```python
from build123d import *

# Parameters (mm, degrees)
F2_DEPTH = 100
F3_W     = 86
F3_H     = 92
F4_DEPTH = 3


# Not quite as in the source:
# - the program builds the solid bodies; features that only make, move or delete a surface that nothing else refers to are left out


with BuildPart() as f2:
    # F0 (on Top) → F2 (new body)
    with BuildSketch(Plane.XY):
        Polygon((-2.3052925244, 0), (87.6947074756, 0), (87.6947074756, 8), (85.6947074756, 8), (85.6947074756, 3), (-0.3052925244, 3), (-0.3052925244, 11), (-59.3052925244, 11), (-59.3052925244, 8), (-2.3052925244, 8), (-2.3052925244, 3), align=None)
    extrude(amount=-F2_DEPTH)

    # F3 (on Front) → F4 (cut)
    with BuildSketch(Plane.XZ):
        with Locations((42.6947074756, -50)):
            Rectangle(F3_W, F3_H)
    extrude(amount=-F4_DEPTH, mode=Mode.SUBTRACT)


solid = f2.part
```
Source: CAD feature listing. Evaluate the final solid. Frame: model axes, mm. A direction names the side the tool comes from. Round coordinates to 2 decimals unless told otherwise and drop trailing zeros. Write each loop counter-clockwise with the first axis right and the second up, starting at its lowest first coordinate (ties: lowest second). Pieces come first, ordered by that corner, then holes. Notation, with made-up numbers: M -25.75,-24 L -2.75,-24 A15 ccw -2.75,-17 Z; hole C 44,8 d6. An arc over 180 degrees is marked long. Answer as a JSON object with one key per item and string values. Group by question number.
(1) Ray query, line 1 (X direction, y = 1.5, z = -17); line 2 (X direction, y = 10.5, z = -64); line 3 (Y direction, x = -12.5, z = -81). Return the intervals inside material, ascending. Write a range as [from, to].
(2) Section query C-C on x = 40. Output: boundary loops of the cut face in (y, z).
(3) Mould query, pull axis Z, two halves, no side actions, for faces 1 (the flat face through (42, 1, -96)), 2 (the flat face through (13.9, 2.7, 0)), 3 (the flat face through (-31, 8, -49)). Classes: +Z half, -Z half, draft (parallel to the pull), parting line (faces both ways), or undercut.
(4) Section query A-A on z = -15.5. Output: boundary loops of the cut face in (x, y).
(5) First-contact query: pin 1 (5 mm diameter, centred on x = -35.5, y = 3.5, fed in from -Z); pin 2 (1.2 mm diameter, centred on x = 45, z = -3, fed in from +Y); pin 3 (1.6 mm diameter, centred on x = 87, z = -26, fed in from +Y); pin 4 (6.5 mm diameter, centred on y = 3, z = -52, fed in from -X). Flat tips, straight axial feed; report the tip coordinate or a pass-through.
(6) Section query D-D on x = -7. Output: boundary loops of the cut face in (y, z), then the cut area to 3 significant figures.
(7) Reachability of faces 4 (the flat face through (-29, 11, -49)), 5 (the flat face through (-2.305, 4, -49)), 6 (the flat face through (43, 3, -98)), 7 (the flat face through (87.695, 4, -49)), 8 (the flat face through (42, 1, -4)) from +Z, -Z, +X, -X, +Y, -Y: full face, straight path, thin tool, end or side. Return the list, or none.
(8) Section query B-B on y = 6.25. Output: boundary loops of the cut face in (x, z), then the cut area to 3 significant figures.
Computed values:
{
 "1": {"line 1": "[-2.31, -0.31], [85.69, 87.69]", "line 2": "[-59.31, -0.31]", "line 3": "[8, 11]"},
 "2": {"outline": "M 0,-100 L 3,-100 L 3,-96 L 0,-96 Z; M 0,-4 L 3,-4 L 3,0 L 0,0 Z"},
 "3": {"face 1": "undercut", "face 2": "+Z half", "face 3": "draft"},
 "4": {"outline": "M -59.31,8 L -2.31,8 L -2.31,0 L -0.31,0 L -0.31,11 L -59.31,11 Z; M 85.69,0 L 87.69,0 L 87.69,8 L 85.69,8 Z"},
 "5": {"pin 1": "through", "pin 2": "y = 3", "pin 3": "y = 8", "pin 4": "x = -2.31"},
 "6": {"outline": "M 8,-100 L 11,-100 L 11,0 L 8,0 Z", "area": "300 mm^2"},
 "7": {"face 4": "+Z, -Z, +X, -X, +Y", "face 5": "+Z, -Z, -X, -Y", "face 6": "+Z, -Z, +Y", "face 7": "+Z, -Z, +X, +Y, -Y", "face 8": "+Y, -Y"},
 "8": {"outline": "M -2.31,-100 L -0.31,-100 L -0.31,0 L -2.31,0 Z; M 85.69,-100 L 87.69,-100 L 87.69,0 L 85.69,0 Z", "area": "400 mm^2"}
}
